Autodesk Inventor part; units mm, degrees
ref_plane "YZ Plane" through (0, 0, 0) normal (1, 0, 0) x (0, 1, 0)
ref_plane "XZ Plane" through (0, 0, 0) normal (0, 1, 0) x (-1, 0, 0)
ref_plane "XY Plane" through (0, 0, 0) normal (0, 0, 1) x (1, 0, 0)
sketch "Sketch1" plane through (0, 0, 0) normal (0, 0, 1) x (1, 0, 0)
  circle A0 centre (0, 0) radius 25.4
  circle A1 centre (-19.05, 0) radius 2.3495
  circle A2 centre (9.525, -16.4978) radius 2.3495
  circle A3 centre (9.525, 16.4978) radius 2.3495
  line L0 (-19.05, 0) -> (0, 0) construction
  dimension "d0" = 50.8
  dimension "d3" = 4.699
  dimension "d6" = 360
  dimension "d8" = 19.05
extrude "Extrusion1" add sketch "Sketch1" along normal blind 6.35
sketch "Sketch2" plane through (0, 0, 6.35) normal (0, 0, 1) x (1, 0, 0)
  arc A0 (2, 7.9524) -> (-2, 7.9524) centre (0, 0) ccw
  arc A1 (-2, 7.9524) -> (-5.8869, 5.7082) centre (0, 0) ccw
  arc A2 (-5.8869, 5.7082) -> (-7.8869, 2.2441) centre (0, 0) ccw
  arc A3 (-7.8869, 2.2441) -> (-7.8869, -2.2441) centre (0, 0) ccw
  arc A4 (-7.8869, -2.2441) -> (-5.8869, -5.7082) centre (0, 0) ccw
  arc A5 (-5.8869, -5.7082) -> (-2, -7.9524) centre (0, 0) ccw
  arc A6 (-2, -7.9524) -> (2, -7.9524) centre (0, 0) ccw
  arc A7 (2, -7.9524) -> (5.8869, -5.7082) centre (0, 0) ccw
  arc A8 (5.8869, -5.7082) -> (7.8869, -2.2441) centre (0, 0) ccw
  arc A9 (7.8869, -2.2441) -> (7.8869, 2.2441) centre (0, 0) ccw
  arc A10 (7.8869, 2.2441) -> (5.8869, 5.7082) centre (0, 0) ccw
  arc A11 (5.8869, 5.7082) -> (2, 7.9524) centre (0, 0) ccw
  arc A12 (2, 9.7469) -> (-2, 9.7469) centre (0, 0) ccw
  line L0 (2, 7.9524) -> (2, 9.7469)
  line L1 (-2, 9.7469) -> (-2, 7.9524)
  line L2 (-5.8869, 5.7082) -> (-7.4411, 6.6055)
  arc A13 (-7.4411, 6.6055) -> (-9.4411, 3.1414) centre (0, 0) ccw
  line L3 (-9.4411, 3.1414) -> (-7.8869, 2.2441)
  line L4 (-7.8869, -2.2441) -> (-9.4411, -3.1414)
  arc A14 (-9.4411, -3.1414) -> (-7.4411, -6.6055) centre (0, 0) ccw
  line L5 (-7.4411, -6.6055) -> (-5.8869, -5.7082)
  line L6 (-2, -7.9524) -> (-2, -9.7469)
  arc A15 (-2, -9.7469) -> (2, -9.7469) centre (0, 0) ccw
  line L7 (2, -9.7469) -> (2, -7.9524)
  line L8 (5.8869, -5.7082) -> (7.4411, -6.6055)
  arc A16 (7.4411, -6.6055) -> (9.4411, -3.1414) centre (0, 0) ccw
  line L9 (9.4411, -3.1414) -> (7.8869, -2.2441)
  line L10 (7.8869, 2.2441) -> (9.4411, 3.1414)
  arc A17 (9.4411, 3.1414) -> (7.4411, 6.6055) centre (0, 0) ccw
  line L11 (7.4411, 6.6055) -> (5.8869, 5.7082)
extrude "Extrusion2" cut sketch "Sketch2" against normal blind 25.4
properties part number "Small Gear Spacer" material "Polycarbonate, Clear"
Input: part model. Units: mm. Frame: model coordinates. Coordinates: 2 decimals unless noted, no trailing zeros. Loops run counter-clockwise (first coordinate to the right, second up) from the corner with the lowest first, then second, coordinate; pieces in that order, holes last.
Q1. Cut plane A-A (x = 0). Output: boundary loops of the cut face in (y, z).
Q2. Cut plane D-D (x = -19.05). Output: boundary loops of the cut face in (y, z).
Q3. Cut plane B-B (y = 0). Output: boundary loops of the cut face in (x, z), then the cut area to 3 significant figures.
Q4. Contact query for flat-ended pins moving along their axis: pin 1 (3 mm diameter, centred on x = 9.52, y = 16.5, fed in from -Z); pin 2 (3 mm diameter, centred on x = -15.5, z = 1.5, fed in from +Y); pin 3 (0.9 mm diameter, centred on y = 9, z = 2.5, fed in from -X); pin 4 (1.4 mm diameter, centred on y = 9, z = 2, fed in from +X). Output: stop coordinate, or through.
Q5. Cut plane C-C (z = 5.5). Give the number of separate pieces and of enclosed holes in the cut face, then the cut area to 3 significant figures.
Q6. Draft query along Y for faces 1 (the face through (8.653, 2.686, 3.219)), 2 (the face through (-6, 6, 0)). Return one class per face: +Y half, -Y half, draft (parallel to the pull), parting line (faces both ways), or undercut.
Q7. Material intervals for line 1 (Y direction, x = -9, z = 1); line 2 (Y direction, x = 9, z = 5.5); line 3 (X direction, y = -2, z = 4.5), sorted ascending.
Working result:
1. outline: (-25.4, 0) - (-9.95, 0) - (-9.95, 6.35) - (-25.4, 6.35) - close; (9.95, 0) - (25.4, 0) - (25.4, 6.35) - (9.95, 6.35) - close
2. outline: (-16.8, 0) - (-2.35, 0) - (-2.35, 6.35) - (-16.8, 6.35) - close; (2.35, 0) - (16.8, 0) - (16.8, 6.35) - (2.35, 6.35) - close
3. outline: (-25.4, 0) - (-21.4, 0) - (-21.4, 6.35) - (-25.4, 6.35) - close; (-16.7, 0) - (-8.2, 0) - (-8.2, 6.35) - (-16.7, 6.35) - close; (8.2, 0) - (25.4, 0) - (25.4, 6.35) - (8.2, 6.35) - close
3. area: 189 mm2
4. pin 1: passes through
4. pin 2: stops at y = 21.19
4. pin 3: stops at x = -23.92
4. pin 4: stops at x = 24.01
5. separate pieces: 1
5. enclosed holes: 4
5. area: 1,720 mm2
6. face 1: undercut
6. face 2: draft
7. line 1: y = -23.75 to -4.24, -2.89 to 2.89, 4.24 to 23.75
7. line 2: y = -23.75 to -18.79, -14.21 to -4.24, -2.89 to 2.89, 4.24 to 14.21, 18.79 to 23.75
7. line 3: x = -25.32 to -20.28, -17.82 to -7.95, 7.95 to 25.32
